Can you work these out from the model? Positions are in its coordinate system, mm. Give positions to 0.01 mm unless a question says otherwise; leave off trailing zeros. Write each loop counter-clockwise with the first axis right and the second up, starting at its lowest first coordinate (ties: lowest second). Pieces come first, ordered by that corner, then holes.
from build123d import *

# Parameters (mm, degrees)
SKETCH1_W                             = 127
SKETCH1_H                             = 76.2
BOSS_EXTRUDE1_DEPTH                   = 6.35
CUT_EXTRUDE1_DEPTH                    = 149.24224263
CUT_EXTRUDE1_DEPTH_BACK               = 149.24224263
SKETCH4_R                             = 3.175
F_1_4_0_25_DIAMETER_HOLE1_D           = 6.35
F_1_4_0_25_DIAMETER_HOLE1_CSINK_D     = 7.62
F_1_4_0_25_DIAMETER_HOLE1_CSINK_ANGLE = 90


with BuildPart() as part:
    # Sketch1 → Boss-Extrude1 (new body)
    with BuildSketch(Plane.XY):
        with Locations((-63.5, 38.1)):
            Rectangle(SKETCH1_W, SKETCH1_H)
    extrude(amount=BOSS_EXTRUDE1_DEPTH)

    # Sketch4 → Cut-Extrude1 (cut, two sides: drawn at the far end of the back side and taken through both)
    with BuildSketch(Plane(origin=(0, 0, 0), x_dir=(-1, 0, 0), z_dir=(0, 0, -1)).offset(-CUT_EXTRUDE1_DEPTH_BACK)):
        with Locations((79.912500047, 64.573038165)):
            Circle(SKETCH4_R)
    extrude(amount=CUT_EXTRUDE1_DEPTH + CUT_EXTRUDE1_DEPTH_BACK, mode=Mode.SUBTRACT)

    # 1/4 (0.25) Diameter Hole1 (through all)
    with Locations(Plane(origin=(0, 0, 0), x_dir=(-1, 0, 0), z_dir=(0, 0, -1))):
        with Locations((116.84, 6.35), (60.96, 6.35)):
            CounterSinkHole(F_1_4_0_25_DIAMETER_HOLE1_D / 2, F_1_4_0_25_DIAMETER_HOLE1_CSINK_D / 2, counter_sink_angle=F_1_4_0_25_DIAMETER_HOLE1_CSINK_ANGLE)


solid = part.part
(1) If I drill on L1, parallel to X at y = 6.35, z = 1.95 (3 decimals); L2, parallel to Y at x = -60.96, z = 3.1 (3 decimals); L3, parallel to X at y = 8, z = 0.5, over which ranges is the centre line in solid material (lowest first)?
Returned:
L1: x = -127 to -120.015, -113.665 to -64.135, -57.785 to 0
L2: y = 0 to 3.175, 9.525 to 76.2
L3: x = -127 to -119.71, -113.97 to -63.83, -58.09 to 0
(2) Imagine slicing it at B-B, the plane x = -116.84. Write out the boundary of the cut face in (y, z) (3 decimals), plus the area to 3 significant figures.
Returned:
outline: (0, 0) - (2.54, 0) - (3.175, 0.635) - (3.175, 6.35) - (0, 6.35) - close; (9.525, 0.635) - (10.16, 0) - (76.2, 0) - (76.2, 6.35) - (9.525, 6.35) - close
area: 443 mm2
(3) If we mould it in two halves opening along X, with no side actions, what happens to faces 1 (the face through (-77.393, 62.641, 3.219)), 2 (the face through (0, 38, 3)), 3 (the face through (-64, 0, 3))? For each: +X half, -X half, draft (parallel to the pull), parting line (faces both ways), or undercut.
Returned:
face 1: undercut
face 2: +X half
face 3: draft
(4) Imagine slicing it at A-A, the plane y = 6.35. Write out the boundary of the cut face in (x, z) (3 decimals).
Returned:
outline: (-127, 0) - (-120.65, 0) - (-120.015, 0.635) - (-120.015, 6.35) - (-127, 6.35) - close; (-113.665, 0.635) - (-113.03, 0) - (-64.77, 0) - (-64.135, 0.635) - (-64.135, 6.35) - (-113.665, 6.35) - close; (-57.785, 0.635) - (-57.15, 0) - (0, 0) - (0, 6.35) - (-57.785, 6.35) - close
(5) Will this pin go through, and if not, where does the flat tip stop? P1, Ø2, axis at x = -25, z = 4.5, coming from the -Y side.
Returned:
P1: stops at y = 0
